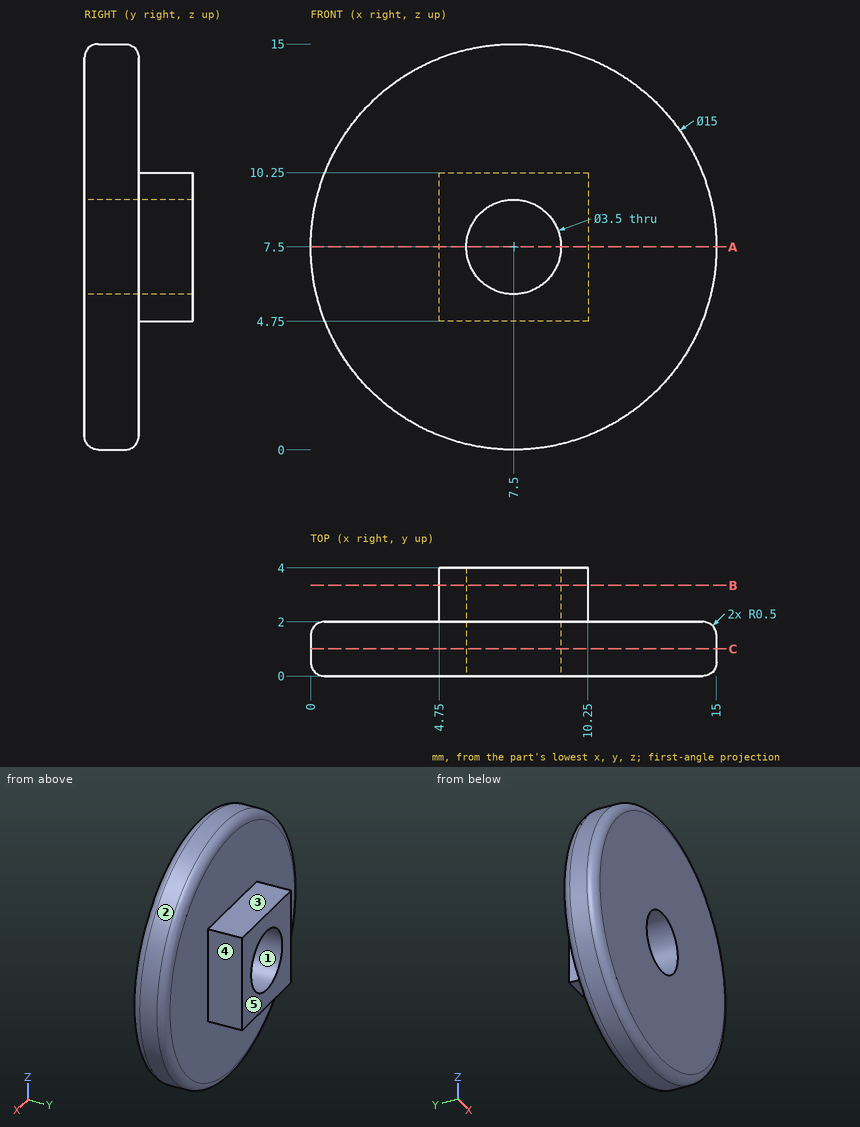
Verification items for this drawing (mm, ordinates from the low corner). A direction names the side the tool comes from. Coordinates: 2 decimals unless noted, no trailing zeros. Order: outer loops, then holes, each group sorted by start corner. A loop starts at its lowest first (then second) coordinate and runs counter-clockwise, first axis right, second up. Notation, with made-up numbers: (-38, 74) -> (-11, 74) arc R14 ccw to (-11, 87) -> close; hole circle Ø8 at (59, 26.5). An arc over 180 degrees is marked (long way). Put each result on its own line as item: value. Start each with the question number.
1. Go/stop test with flat-tipped pins: pin 1 Ø1 at (x, z) = (5.5, 12.5) entering from -Y; pin 2 Ø1.6 at (x, y) = (8.5, 3.5) entering from +Z; pin 3 Ø1.5 at (y, z) = (2.5, 11.5) entering from +X; pin 4 Ø3 at (x, z) = (7.5, 7.5) entering from -Y. Record where each tip stops, or that it passes through.
2. Cross-section at C-C, the plane y = 1. Record the boundary of the cut face in (x, z), then the cut area to 3 significant figures.
3. Material ranges on L1, parallel to Z at x = 7.5, y = 3.2; L2, parallel to Y at x = 2.75, z = 10.75; L3, parallel to Z at x = 9.5, y = 3.55, recorded low to high. Write a range as [from, to].
4. Cross-section at A-A, the plane z = 7.5. Record the boundary of the cut face in (x, y).
5. Cross-section at B-B, the plane y = 3.35. Record the boundary of the cut face in (x, z), then the cut area to 3 significant figures.
6. Mould release check, pull along X, two halves, no side actions. Record for the marked faces 1, 2 and 3: released by +X, released by -X, zero draft, split by the parting line, or undercut.
7. Access from +Z, -Z, +X, -X, +Y, -Y to the whole of each face (thin tool, end or side, straight path). Record for the marked faces 4 and 5.
Computed:
1. pin 1: y = 0
1. pin 2: z = 10.25
1. pin 3: x = 13.9
1. pin 4: through
2. outline: circle Ø15 at (7.5, 7.5); hole circle Ø3.5 at (7.5, 7.5)
2. area: 167 mm2
3. L1: [4.75, 5.75], [9.25, 10.25]
3. L2: [0, 2]
3. L3: [4.75, 10.25]
4. outline: (0, 0.5) arc R0.5 ccw to (0.5, 0) -> (5.75, 0) -> (5.75, 4) -> (4.75, 4) -> (4.75, 2) -> (0.5, 2) arc R0.5 ccw to (0, 1.5) -> close; (9.25, 0) -> (14.5, 0) arc R0.5 ccw to (15, 0.5) -> (15, 1.5) arc R0.5 ccw to (14.5, 2) -> (10.25, 2) -> (10.25, 4) -> (9.25, 4) -> close
5. outline: (4.75, 4.75) -> (10.25, 4.75) -> (10.25, 10.25) -> (4.75, 10.25) -> close; hole circle Ø3.5 at (7.5, 7.5)
5. area: 20.6 mm2
6. face 1: undercut
6. face 2: split by the parting line
6. face 3: zero draft
7. face 4: +Z, -Z, +X, +Y
7. face 5: +Z, -Z, +X, -X, +Y
